Design review of the part built by this model. Coordinates are the model's own, in mm. Face numbers are marked on the shaded views. A direction names the side the tool comes from. Coordinates: 2 decimals unless noted, no trailing zeros. Loops run counter-clockwise (first coordinate to the right, second up) from the corner with the lowest first, then second, coordinate; pieces in that order, holes last. Notation, with made-up numbers: (41, -9.75) - (54, -9.75) arc R23 ccw to (54, 25.25) - close; hole circle Ø3 at (15.5, 86.5). An arc over 180 degrees is marked (long way). Use one line per item in the form item = value. Start each with the question number.
(1) Add section A-A (x = 2.75). State the section outline as (y, z) points, plus the area to 3 significant figures.
(2) The part is to be moulded in two halves that separate along Z. For the marked faces 3, 4 and 5, say which applies: pulls with the +Z half, pulls with the -Z half, needs draft (parallel to the pull), parting line crosses it, or undercut.
(3) Clearance check with flat-ended pins moving along their axes: pin 1 Ø3 at (x, y) = (9, 2.5) entering from -Z; pin 2 Ø2 at (x, z) = (8.5, -2) entering from +Y; pin 3 Ø2 at (x, y) = (7.5, -1) entering from -Z. State where each tip first meets the part, or that it passes through.
(4) For L1, parallel to Z at x = 0.5, y = 1; L2, parallel to Y at x = 1, z = 0.25; L3, parallel to X at y = 0.5, z = -2.5, list the stretches that pass through material, from the lowest coordinate up.
(5) Tool access review of the marked faces 1 and 2: name each direction out of +Z, -Z, +X, -X, +Y, -Y from which nothing blocks a thin tool from reaching the whole face with its end or side.
```python
from build123d import *

# Parameters (mm, degrees)
FILLET2_R        = 0.2
LPATTERN10_COUNT = 20
LPATTERN10_PITCH = 0.25


with BuildPart() as part:
    # Sketch1 → Base (revolve)
    with BuildSketch(Plane(origin=(0, 0, 0), x_dir=(1, 0, 0), z_dir=(0, 1, 0))):
        Polygon((1.7, 1.5), (12, 1.5), (12, 0), (0, 0), (0, 3), (0.2, 3), align=None)
    revolve(axis=Axis((-6.506452013, 0, 0), (1, 0, 0)))

    # Sketch3 → Cut-Revolve1 (revolve, cut)
    with BuildSketch(Plane.XY):
        Polygon((12.15755877, 0), (12.15755877, 20), (0.452994616, 20), (12, 0), align=None)
    revolve(axis=Axis((4.883468835, 0, 0), (1, 0, 0)), mode=Mode.SUBTRACT)

    # Fillet2
    fillet2_edges = [part.edges().sort_by_distance(p)[0] for p in [
        (1.7, 0, 1.5),
    ]]
    fillet(fillet2_edges, radius=FILLET2_R)

    # Sketch2 → Cut-Loft1 section 0
    with BuildSketch(Plane(origin=(0, -0.680816871, 0.306758275), x_dir=(0, 0, 1), z_dir=(-1, 0, 0)), mode=Mode.PRIVATE) as cut_loft1_s0:
        Polygon((-0.686758275, 1.060816871), (-2.206758275, 1.060816871), (-2.206758275, 0.300816871), (-0.686758275, 0.300816871), (-0.686758275, -1.219183129), (0.073241725, -1.219183129), (0.073241725, 0.300816871), (1.593241725, 0.300816871), (1.593241725, 1.060816871), (0.073241725, 1.060816871), (0.073241725, 2.580816871), (-0.686758275, 2.580816871), align=None)
    loft([cut_loft1_s0.sketch, Vertex(1.95, 0, 0)], mode=Mode.SUBTRACT)

    # Sketch5 → Cut-Revolve10 (revolve, cut)
    with BuildSketch(Plane.XY):
        Polygon((7, 1.7), (7.125, 1.7), (7.125, 1.5), (7.0625, 1.391746825), (7, 1.5), align=None)
    cut_revolve10 = revolve(axis=Axis((10.774329131, 0, 0), (-1, 0, 0)), mode=Mode.SUBTRACT)

    # LPattern10: Cut-Revolve10 ×20
    with Locations(*[(i * LPATTERN10_PITCH, 0, 0) for i in range(1, LPATTERN10_COUNT)]):
        add(cut_revolve10, mode=Mode.SUBTRACT)


solid = part.part
```
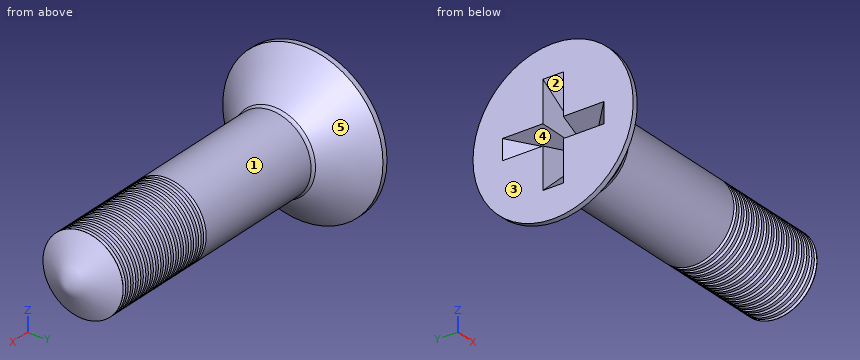
Computed values:
q1.outline = circle Ø3 at (0, 0)
q1.area = 7.07 mm^2
q2.face_3 = needs draft
q2.face_4 = undercut
q2.face_5 = parting line crosses it
q3.pin_1 = -1.12
q3.pin_2 = 1.12
q3.pin_3 = -1.5
q4.L1 = -2.51 to -0.28, 0.28 to 2.51
q4.L2 = -2.19 to -0.19, 0.19 to 2.19
q4.L3 = 0 to 0.65
q5.face_1 = +X
q5.face_2 = -X
